Here's the drawing with two shaded views (mm, measured from the low corner). I have some questions. A direction names the side the tool comes from. Round coordinates to 2 decimals unless told otherwise and drop trailing zeros. Order: outer loops, then holes, each group sorted by start corner. A loop starts at its lowest first (then second) coordinate and runs counter-clockwise, first axis right, second up.
Q1. If we section it at D-D (y = 63.5): Please give me the cut outline in (x, z).
Q2. Will these pins go through, and if not, where does the flat tip stop? P1, Ø23.5, axis at x = 25.4, y = 42.18, coming from the -Z side; P2, Ø1, axis at x = 19, z = 20.5, coming from the +Y side; P3, Ø8, axis at x = 44, z = 16.5, coming from the -Y side; P4, Ø5, axis at x = 41, y = 45, coming from the -Z side.
Q3. If we section it at A-A (x = 25.4): Please give me the cut outline in (y, z).
Q4. If we section it at B-B (y = 36): Please give me the cut outline in (x, z).
Q5. For the marked faces 1 and 2, which set-ups out of +Z, -Z, +X, -X, +Y, -Y let a thin tool reach every point of the face, with its end or its side?
Q6. We'd pull the mould along X, two halves only. Please class the marked faces 3, 4, 5 and 6: pulls with the +X half, pulls with the -X half, needs draft (parallel to the pull), parting line crosses it, or undercut.
Q7. If I drill on line 1 (Y direction, x = 25.4, z = 34); line 2 (Z direction, x = 31.5, y = 24); line 3 (Y direction, x = 17, z = 14.5), over which ranges is the centre line in solid material (lowest first)?
Q8. If we section it at C-C (z = 12): Please give me the cut outline in (x, y), plus the area to 3 significant figures.
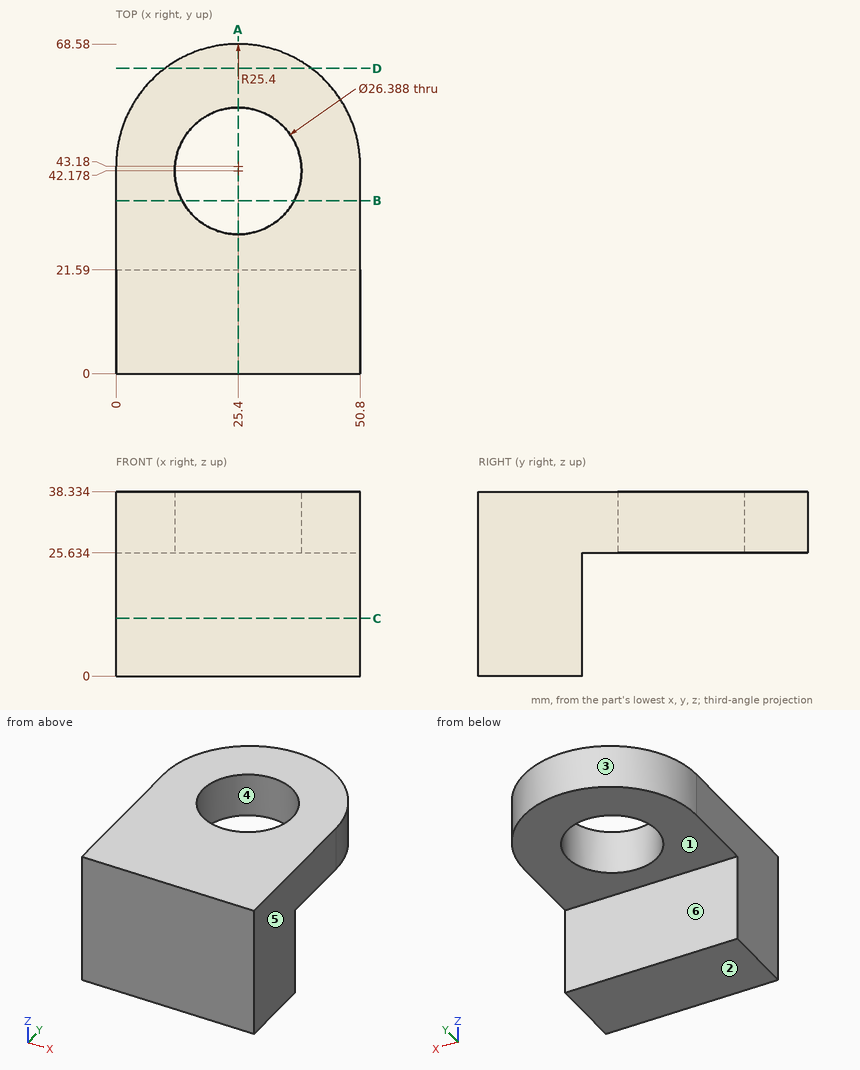
Solution:
1. outline: (10.16, 25.63) - (40.64, 25.63) - (40.64, 38.33) - (10.16, 38.33) - close
2. P1: passes through
2. P2: stops at y = 21.59
2. P3: stops at y = 0
2. P4: stops at z = 25.63
3. outline: (0, 0) - (21.59, 0) - (21.59, 25.63) - (28.98, 25.63) - (28.98, 38.33) - (0, 38.33) - close; (55.37, 25.63) - (68.58, 25.63) - (68.58, 38.33) - (55.37, 38.33) - close
4. outline: (0, 25.63) - (13.74, 25.63) - (13.74, 38.33) - (0, 38.33) - close; (37.06, 25.63) - (50.8, 25.63) - (50.8, 38.33) - (37.06, 38.33) - close
5. face 1: -Z, +X, -X, +Y
5. face 2: -Z, +X, -X, +Y, -Y
6. face 3: parting line crosses it
6. face 4: undercut
6. face 5: pulls with the +X half
6. face 6: needs draft
7. line 1: y = 0 to 28.98, 55.37 to 68.58
7. line 2: z = 25.63 to 38.33
7. line 3: y = 0 to 21.59
8. outline: (0, 0) - (50.8, 0) - (50.8, 21.59) - (0, 21.59) - close
8. area: 1,100 mm2
